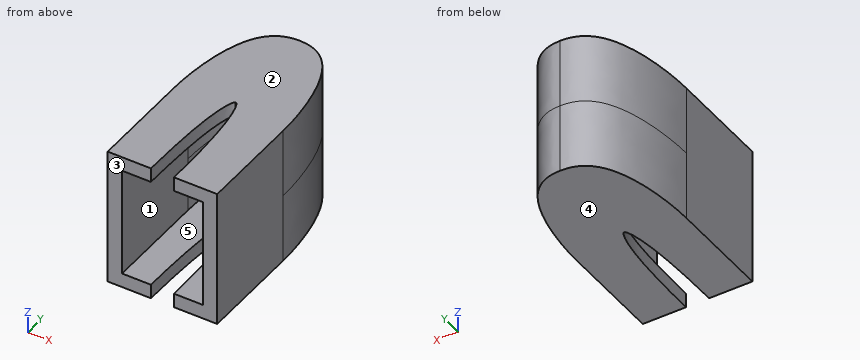
Autodesk Fusion 360 part; units mm, degrees
sketch "Skizze1" plane through (0, 0, 0) normal (0, 0, 1) x (1, 0, 0)
  line L0 (0, 0) -> (0, 35)
  line L1 (7, 0) -> (9.5, 0)
  line L2 (9.5, 0) -> (9.5, 18)
  line L3 (9.5, 18) -> (7, 18) construction
  line L4 (7, 18) -> (7, 0)
  spline S0 degree 5 poles (0, 35) (0.73, 35) (2.063, 34.7613) (3.6816, 33.688) (5.1796, 31.0566) (6.2948, 26.6703) (6.7786, 22.9675) (6.9597, 20.3756) (7, 18.7712) (7, 18) knots 0 0 0 0 0 0 0.2 0.4 0.6 0.8 1 1 1 1 1 1
  spline S1 degree 5 poles (0, 37.5) (0.9879, 37.5) (2.7924, 37.2385) (4.9853, 36.0627) (7.0185, 33.1717) (8.5367, 28.287) (9.1974, 24.0454) (9.445, 20.9552) (9.5, 18.9722) (9.5, 18) knots 0 0 0 0 0 0 0.2 0.4 0.6 0.8 1 1 1 1 1 1
  line L5 (0, 37.5) -> (0, 35)
  line L6 (-2.5, 37.5) -> (2.5, 37.5)
  line L7 (-1.5, 35) -> (1.5, 35)
  line L8 (7, 20) -> (7, 16)
  line L9 (9.5, 21) -> (9.5, 15)
  line L10 (0, 0) -> (7, 0)
  circle A0 centre (0, 16) radius 1
  line L11 (1, 16) -> (1, 0)
  line L12 (0, 0) -> (0, -5) construction
  line L13 (0, 37.5) -> (0, 35)
  line L14 (-1, 16) -> (-1, 0)
  line L15 (-7, 20) -> (-7, 16)
  circle A1 centre (0, 16) radius 1
  spline S2 degree 5 poles (0, 37.5) (-0.9879, 37.5) (-2.7924, 37.2385) (-4.9853, 36.0627) (-7.0185, 33.1717) (-8.5367, 28.287) (-9.1974, 24.0454) (-9.445, 20.9552) (-9.5, 18.9722) (-9.5, 18) knots 0 0 0 0 0 0 0.2 0.4 0.6 0.8 1 1 1 1 1 1
  line L16 (2.5, 37.5) -> (-2.5, 37.5)
  line L17 (-9.5, 21) -> (-9.5, 15)
  line L18 (-9.5, 21) -> (-9.5, 15)
  line L19 (0, 0) -> (-7, 0)
  line L20 (-9.5, 0) -> (-9.5, 18)
  line L21 (-9.5, 18) -> (-7, 18) construction
  spline S3 degree 5 poles (0, 35) (-0.73, 35) (-2.063, 34.7613) (-3.6816, 33.688) (-5.1796, 31.0566) (-6.2948, 26.6703) (-6.7786, 22.9675) (-6.9597, 20.3756) (-7, 18.7712) (-7, 18) knots 0 0 0 0 0 0 0.2 0.4 0.6 0.8 1 1 1 1 1 1
  line L22 (1.5, 35) -> (-1.5, 35)
  line L23 (-7, 20) -> (-7, 16)
  line L24 (-7, 0) -> (-9.5, 0)
  line L25 (-7, 18) -> (-7, 0)
  line L26 (0, 0) -> (0, 35)
  line L27 (1.5, 35) -> (-1.5, 35)
  line L28 (2.5, 37.5) -> (-2.5, 37.5)
  dimension "d1" = 18
  dimension "d2" = 5
  dimension "d3" = 3
  dimension "d4" = 4
  dimension "d5" = 6
  dimension "d6" = 7
  dimension "d7" = 35
  dimension "d8" = 2.5
  dimension "d9" = 16
  dimension "d10" = 2
extrude "Extrusion1" add sketch "Skizze1" along normal mid plane 24
shell "Schale1" thickness 2.5 removed faces 1 at (3.1667, 0, 4)
sketch "Skizze2" plane through (0, 0, 12) normal (0, 0, 1) x (1, 0, 0)
  line L0 (-9.5, 0) -> (9.5, 0)
  line L1 (9.5, 0) -> (9.5, 18)
  spline S0 degree 5 poles (9.5, 18) (9.5, 18.9722) (9.445, 20.9552) (9.1974, 24.0454) (8.5367, 28.287) (7.0185, 33.1717) (4.9853, 36.0627) (2.7924, 37.2385) (0.9879, 37.5) (0, 37.5) knots -1 -1 -1 -1 -1 -1 -0.8 -0.6 -0.4 -0.2 0 0 0 0 0 0
  spline S1 degree 5 poles (0, 37.5) (-0.9879, 37.5) (-2.7924, 37.2385) (-4.9853, 36.0627) (-7.0185, 33.1717) (-8.5367, 28.287) (-9.1974, 24.0454) (-9.445, 20.9552) (-9.5, 18.9722) (-9.5, 18) knots 0 0 0 0 0 0 0.2 0.4 0.6 0.8 1 1 1 1 1 1
  line L2 (-9.5, 18) -> (-9.5, 0)
  spline S2 degree 5 poles (-2, 0) (-2, 2.2036) (-1.9635, 6.2369) (-1.7993, 11.1651) (-1.4009, 15.6523) (-0.8096, 18.6119) (-0.3036, 19.8562) (-0.0021, 20.1554) (0.2998, 19.8561) (0.8069, 18.6119) (1.3996, 15.6524) (1.7989, 11.1652) (1.9634, 6.237) (2, 2.2037) (2, 0) knots 0 0 0 0 0 0 0.1 0.2 0.3 0.4 0.5 0.6 0.7 0.8 0.9 1 1 1 1 1 1
  line L3 (0, 0) -> (-0.002, 20) construction
  line L4 (-0.102, 20) -> (0.098, 20)
  line L5 (2, 5) -> (2, -5)
  line L6 (-2, -5) -> (-2, 5)
  point P0 (-0.002, 20)
  dimension "d14" = 4
  dimension "d15" = 10
  dimension "d16" = 0.2
  dimension "d17" = 20
extrude "Extrusion2" cut sketch "Skizze2" against normal blind 24 contours L0 S2
Model file for the job. Use its own axes, mm. Face numbers are marked on the shaded views. A direction names the side the tool comes from. Round coordinates to 2 decimals unless told otherwise and drop trailing zeros. Write each question's results on one line, items separated by ' | '.
(1) 3-axis set-ups, long thin cutter, end or side, ignore diameter. For the marked faces 1 and 2: which of +Z, -Z, +X, -X, +Y, -Y reach the whole face in a straight line?
Answer below:
face 1: -Y | face 2: +Z, +X, -X, +Y, -Y
(2) Mould opens along Z. For the marked faces 3, 4 and 5 say: released by +Z, released by -Z, zero draft, split by the parting line, or undercut.
Answer below:
face 3: zero draft | face 4: released by -Z | face 5: undercut
(3) Wall check: L1, parallel to Z at x = -1.5, y = 33; L2, parallel to X at y = 2.5, z = -0.5; L3, parallel to X at y = 3.5, z = -10.5. Give the ranges that are in metal, low to high.
Answer below:
L1: z = -12 to -9.5, 9.5 to 12 | L2: x = -9.5 to -7, 7 to 9.5 | L3: x = -9.5 to -1.98, 1.98 to 9.5
(4) Pin check, flat tips, straight feed: pin 1 (6 mm diameter, centred on x = 5.5, z = -3.5, fed in from +Y); pin 2 (1.5 mm diameter, centred on x = 2.5, z = -5, fed in from -Y). Stop position of each tip, or through.
Answer below:
pin 1: stops at y = 37.09 | pin 2: stops at y = 33.66
